For this review, take the finished solid that the model builds, in its own axes (mm). Round coordinates to 2 decimals unless told otherwise and drop trailing zeros. Write each loop counter-clockwise with the first axis right and the second up, starting at its lowest first coordinate (ties: lowest second). Pieces come first, ordered by that corner, then holes.
Autodesk Inventor part; units mm, degrees
ref_plane "YZ Plane" through (0, 0, 0) normal (1, 0, 0) x (0, 1, 0)
ref_plane "XZ Plane" through (0, 0, 0) normal (0, 1, 0) x (-1, 0, 0)
ref_plane "XY Plane" through (0, 0, 0) normal (0, 0, 1) x (1, 0, 0)
sketch "Sketch1" plane through (0, 0, 0) normal (0, 0, 1) x (1, 0, 0)
  line L0 (0, 0) -> (63.5, 0)
  line L1 (63.5, 0) -> (63.5, -69.85)
  line L2 (63.5, -69.85) -> (0, -69.85)
  line L3 (0, -69.85) -> (0, 0)
  dimension "d0" = 63.5
  dimension "d1" = 69.85
  dimension "d2" = 63.5
extrude "Extrusion1" add sketch "Sketch1" along normal blind 50.8
sketch "Sketch2" plane through (0, 0, 50.8) normal (0, 0, 1) x (1, 0, 0)
  line L0 (0, -69.85) -> (63.5, -69.85)
  circle A0 centre (31.75, -69.85) radius 31.75
  circle A1 centre (31.75, -69.85) radius 15.875
  point P0 (0, 0)
  dimension "d5" = 31.75
extrude "Extrusion2" add sketch "Sketch2" along normal blind 9.525 and the other way blind 60.325 contours A1 L0 A0 | L0 A0 A1
sketch "Sketch3" plane through (63.5, 0, 50.8) normal (1, 0, 0) x (0, 0, -1)
  point P0 (50.8, 0)
sketch "Sketch4" plane through (0, 0, 50.8) normal (0, 0, 1) x (1, 0, 0)
  line L0 (47.625, -69.85) -> (15.875, -69.85)
  circle A0 centre (31.75, -69.85) radius 15.875
  point P0 (0, 0)
  dimension "d10" = 31.75
sketch "Sketch5" plane through (0, 0, 50.8) normal (0, 0, 1) x (1, 0, 0)
  point P0 (0, 0)
extrude "Extrusion3" cut sketch "Sketch4" against normal through all
sketch "Sketch6" plane through (63.5, 0, 50.8) normal (1, 0, 0) x (0, 0, -1)
  line L0 (50.8, 0) -> (0, 0)
  circle A0 centre (25.4, 0) radius 25.4
  dimension "d13" = 50.8
extrude "Extrusion4" add sketch "Sketch6" along normal blind 6.35 and the other way blind 69.85
sketch "Sketch7" plane through (69.85, 0, 25.4) normal (1, 0, 0) x (0, 0, -1)
  circle A0 centre (0, 0) radius 12.7
  point P0 (25.4, 0)
  dimension "d18" = 25.4
extrude "Extrusion5" cut sketch "Sketch7" against normal through all
properties part number "HW 6 Part 5"
(1) We need section A-A, the plane x = 31.75. Give the boundary of the cut face in (y, z) (3 decimals), and give its area (3 significant figures).
Geometry check:
outline: (-101.6, -9.525) - (-85.725, -9.525) - (-85.725, 60.325) - (-101.6, 60.325) - close; (-53.975, -9.525) - (-38.1, -9.525) - (-38.1, 0) - (0, 0) arc R25.4 ccw to (0, 50.8) - (-38.1, 50.8) - (-38.1, 60.325) - (-53.975, 60.325) - close; hole circle Ø25.4 at (0, 25.4)
area: 4,660 mm2
(2) We need section B-B, the plane z = 25.4. Give the boundary of the cut face in (x, y) (3 decimals).
Geometry check:
outline: (-6.35, -25.4) - (0, -25.4) - (0, -69.85) arc R31.75 ccw to (63.5, -69.85) - (63.5, -25.4) - (69.85, -25.4) - (69.85, -12.7) - (-6.35, -12.7) - close; (-6.35, 12.7) - (69.85, 12.7) - (69.85, 25.4) - (-6.35, 25.4) - close; hole circle Ø31.75 at (31.75, -69.85)
(3) We need section D-D, the plane z = 43. Give the boundary of the cut face in (x, y) (3 decimals).
Geometry check:
outline: (-6.35, -18.314) - (0, -18.314) - (0, -69.85) arc R31.75 ccw to (63.5, -69.85) - (63.5, -18.314) - (69.85, -18.314) - (69.85, 18.314) - (-6.35, 18.314) - close; hole circle Ø31.75 at (31.75, -69.85)
(4) For line 1 along Y through (x, z) = (29, 25.4) (3 decimals); line 2 along Y through (x, z) = (31, 28); line 3 along X through (y, z) = (-69, 10), list the stretches that pass through material, from the lowest coordinate up.
Geometry check:
line 1: y = -101.481 to -85.485, -54.215 to -12.7, 12.7 to 25.4
line 2: y = -101.59 to -85.71, -53.99 to -12.43, 12.43 to 25.27
line 3: x = 0 to 15.9, 47.6 to 63.5
(5) Mouldability with a two-part tool opening along X and no side actions: class faces 1 (the face through (32.283, 25.184, 28.707)), 2 (the face through (-6.35, 12, 20)), 3 (the face through (28.309, -85.347, 25.889)) as pulls with the +X half, pulls with the -X half, needs draft (parallel to the pull), parting line crosses it, or undercut.
Geometry check:
face 1: needs draft
face 2: pulls with the -X half
face 3: undercut
(6) For pin 1 Ø1.5 at (x, z) = (35, 21.5) entering from +Y; pin 2 Ø2 at (y, z) = (-35.5, 13) entering from +X; pin 3 Ø4 at (x, y) = (28, -2) entering from +Z, all flat-tipped, find the tip position at first contact; note any pin that passes through.
Geometry check:
pin 1: stops at y = 25.2
pin 2: stops at x = 63.5
pin 3: stops at z = 50.8
(7) We need section C-C, the plane y = -2.5. Give the boundary of the cut face in (x, z), and give its area (3 significant figures).
Geometry check:
outline: (-6.35, 0.12) - (0, 0.12) - (0, 0) - (63.5, 0) - (63.5, 0.12) - (69.85, 0.12) - (69.85, 12.95) - (-6.35, 12.95) - close; (-6.35, 37.85) - (69.85, 37.85) - (69.85, 50.68) - (63.5, 50.68) - (63.5, 50.8) - (0, 50.8) - (0, 50.68) - (-6.35, 50.68) - close
area: 1,970 mm2
